Geometry: final body of the model. Coordinates: model frame, mm. A direction names the side the tool comes from. Give positions to 0.01 mm unless a question says otherwise; leave off trailing zeros. Write each loop counter-clockwise with the first axis right and the second up, starting at its lowest first coordinate (ties: lowest second). Pieces come first, ordered by that corner, then holes.
```python
from build123d import *

# Parameters (mm, degrees)
F0_W     = 80
F0_H     = 80
F1_DEPTH = 25.4
F2_W     = 40
F2_H     = 40
F3_DEPTH = 25.4
F5_D     = 15
F6_R     = 5
F7_R     = 5


with BuildPart() as f1:
    # F0 (on Top) → F1 (new body)
    with BuildSketch(Plane.XY):
        Rectangle(F0_W, F0_H)
    extrude(amount=F1_DEPTH)

    # F2 (on face) → F3 (cut)
    with BuildSketch(Plane.XY.offset(25.4)):
        Rectangle(F2_W, F2_H)
    extrude(amount=-F3_DEPTH, mode=Mode.SUBTRACT)

    # F5 (through all)
    with Locations(Plane.XY.offset(25.4)):
        with Locations((-30, -30), (30, -30), (30, 30), (-30, 30)):
            Hole(F5_D / 2)

    # F6
    f6_edges = [f1.edges().sort_by_distance(p)[0] for p in [
        (40, -40, 12.7),
        (-40, -40, 12.7),
        (40, 40, 12.7),
        (-40, 40, 12.7),
    ]]
    fillet(f6_edges, radius=F6_R)

    # F7
    f7_edges = [f1.edges().sort_by_distance(p)[0] for p in [
        (-20, 20, 12.7),
        (-20, -20, 12.7),
        (20, 20, 12.7),
        (20, -20, 12.7),
    ]]
    fillet(f7_edges, radius=F7_R)


solid = f1.part
```
Item 1: Section A-A, the plane x = 30. Return the cut outline in (y, z), plus the area to 3 significant figures.
Found:
outline: (-40, 0) - (-37.5, 0) - (-37.5, 25.4) - (-40, 25.4) - close; (-22.5, 0) - (22.5, 0) - (22.5, 25.4) - (-22.5, 25.4) - close; (37.5, 0) - (40, 0) - (40, 25.4) - (37.5, 25.4) - close
area: 1,270 mm2
Item 2: Reachability of faces 1 (the face through (19, 18, 13)), 2 (the face through (38, -39, 13)) from +Z, -Z, +X, -X, +Y, -Y: full face, straight path, thin tool, end or side. Return the list, or none.
Found:
face 1: +Z, -Z
face 2: +Z, -Z, +X, -Y
Item 3: Section C-C, the plane z = 21.5. Return the cut outline in (x, y), plus the area to 3 significant figures.
Found:
outline: (-40, -35) arc R5 ccw to (-35, -40) - (35, -40) arc R5 ccw to (40, -35) - (40, 35) arc R5 ccw to (35, 40) - (-35, 40) arc R5 ccw to (-40, 35) - close; hole circle Ø15 at (-30, -30); hole circle Ø15 at (-30, 30); hole (-20, -15) arc R5 ccw to (-15, -20) - (15, -20) arc R5 ccw to (20, -15) - (20, 15) arc R5 ccw to (15, 20) - (-15, 20) arc R5 ccw to (-20, 15) - close; hole circle Ø15 at (30, -30); hole circle Ø15 at (30, 30)
area: 4,090 mm2
Item 4: Pull-direction query (Y, two-part tool) for faces 3 (the face through (0, -20, 13)), 4 (the face through (0, 40, 13)), 5 (the face through (-39, -38, 13)), 6 (the face through (31.63, 22.68, 12.52)); classes: +Y half, -Y half, draft (parallel to the pull), parting line (faces both ways), or undercut.
Found:
face 3: undercut
face 4: +Y half
face 5: -Y half
face 6: undercut
Item 5: Section D-D, the plane x = 16. Return the cut outline in (y, z).
Found:
outline: (-40, 0) - (-19.9, 0) - (-19.9, 25.4) - (-40, 25.4) - close; (19.9, 0) - (40, 0) - (40, 25.4) - (19.9, 25.4) - close
Item 6: Pin query (flat end, axial travel): pin 1 Ø13.5 at (x, y) = (-30, -30) entering from +Z; pin 2 Ø19.5 at (x, y) = (30, -30) entering from +Z. Return the tip coordinate at first contact, or that it passes through.
Found:
pin 1: passes through
pin 2: stops at z = 25.4
Item 7: Line query: L1, parallel to Y at x = -30, z = 20; L2, parallel to Y at x = 0, z = 15.5; L3, parallel to X at y = 30.5, z = 11.75. Output: solid intervals per line, ascending.
Found:
L1: y = -40 to -37.5, -22.5 to 22.5, 37.5 to 40
L2: y = -40 to -20, 20 to 40
L3: x = -40 to -37.48, -22.52 to 22.52, 37.48 to 40
